Build history of the part. All positions in model axes, mm. Face numbers are marked on the shaded views. A direction names the side the tool comes from. Give positions to 0.01 mm unless a question says otherwise; leave off trailing zeros. Loops run counter-clockwise (first coordinate to the right, second up) from the corner with the lowest first, then second, coordinate; pieces in that order, holes last. Notation, with made-up numbers: M -2.5,5.5 L 13.5,5.5 A19 ccw 13.5,34.5 Z; hole C 0.25,83.5 d10. An arc over 180 degrees is marked long. Answer as a JSON object with one key per item and string values. Group by question number.
1. Drill centre lines: line 1 along X through (y, z) = (21.5, -1.3); line 2 along Y through (x, z) = (4.5, -2.3); line 3 along Y through (x, z) = (-6.75, -2.1). Where is each one in solid material? Low to high. Write a range as [from, to].
2. Slice it at A-A (x = 0). List the corners of the cut face in (y, z), then the cut area to 4 significant figures.
3. Slice it at B-B (y = 49.5). List the corners of the cut face in (x, z).
4. Slice it at C-C (z = 0.1). List the corners of the cut face in (x, y), then the cut area to 3 significant figures.
5. Drop flat-ended pins along their axis: pin 1 Ø1 at (x, y) = (4.5, 65) entering from -Z; pin 2 Ø4.5 at (x, y) = (-1, 83) entering from +Z. Give the stop position or say it passes through.
6. Mould opens along Y. For the marked faces 3 and 4 say: released by +Y, released by -Y, zero draft, split by the parting line, or undercut.
7. 3-axis set-ups, long thin cutter, end or side, ignore diameter. For the marked faces 1 and 2: which of +Z, -Z, +X, -X, +Y, -Y reach the whole face in a straight line?
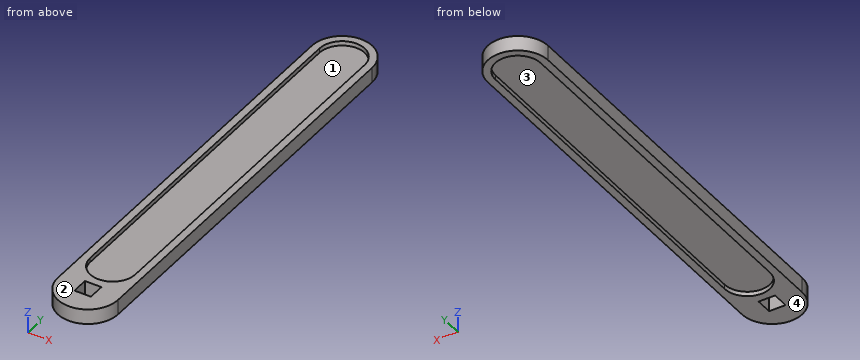
from build123d import *

# Parameters (mm, degrees)
EXTRUDE_1_DEPTH = 1
SKETCH_2_W      = 5.5
SKETCH_2_H      = 5.5
EXTRUDE_2_DEPTH = 2.5


with BuildPart() as part:
    # 草图1 → 凸台-拉伸1 (new body, symmetric)
    with BuildSketch(Plane.XY):
        with BuildLine():
            Line((-7.5, 0), (-7.5, 120))
            ThreePointArc((-7.5, 120), (0, 127.5), (7.5, 120))
            Line((7.5, 120), (7.5, 0))
            ThreePointArc((7.5, 0), (0, -7.5), (-7.5, 0))
        make_face()
    extrude(amount=EXTRUDE_1_DEPTH, both=True)

    # 草图2 → 凸台-拉伸2 (add, symmetric)
    with BuildSketch(Plane.XY):
        with BuildLine():
            Line((-10, 0), (-10, -13))
            ThreePointArc((-10, -13), (0, -23), (10, -13))
            Line((10, -13), (10, 0))
            Line((10, 0), (10, 120))
            ThreePointArc((10, 120), (0, 130), (-10, 120))
            Line((-10, 120), (-10, 0))
        make_face()
        with Locations((0, -13)):
            Rectangle(SKETCH_2_W, SKETCH_2_H, mode=Mode.SUBTRACT)
        with BuildLine():
            Line((-7.5, 120), (-7.5, 0))
            ThreePointArc((-7.5, 0), (0, -7.5), (7.5, 0))
            Line((7.5, 0), (7.5, 120))
            ThreePointArc((7.5, 120), (0, 127.5), (-7.5, 120))
        make_face(mode=Mode.SUBTRACT)
    extrude(amount=EXTRUDE_2_DEPTH, both=True)


solid = part.part
Established:
{
 "1": {"line 1": "x = [-10, -7.5], [7.5, 10]", "line 2": "y = [-21.93, -6], [126, 128.93]", "line 3": "y = [-20.38, -3.27], [123.27, 127.38]"},
 "2": {"outline": "M -23,-2.5 L -15.75,-2.5 L -15.75,2.5 L -23,2.5 Z; M -10.25,-2.5 L -7.5,-2.5 L -7.5,-1 L 127.5,-1 L 127.5,-2.5 L 130,-2.5 L 130,2.5 L 127.5,2.5 L 127.5,1 L -7.5,1 L -7.5,2.5 L -10.25,2.5 Z", "area": "332.5 mm^2"},
 "3": {"outline": "M -10,-2.5 L -7.5,-2.5 L -7.5,-1 L 7.5,-1 L 7.5,-2.5 L 10,-2.5 L 10,2.5 L 7.5,2.5 L 7.5,1 L -7.5,1 L -7.5,2.5 L -10,2.5 Z"},
 "4": {"outline": "M -10,-13 A10 ccw 10,-13 L 10,120 A10 ccw -10,120 Z; hole M -2.75,-15.75 L 2.75,-15.75 L 2.75,-10.25 L -2.75,-10.25 Z", "area": "2,940 mm^2"},
 "5": {"pin 1": "stops at z = -1", "pin 2": "stops at z = 1"},
 "6": {"face 3": "undercut", "face 4": "zero draft"},
 "7": {"face 1": "+Z", "face 2": "+Z, +X, -X, +Y, -Y"}
}
